Could you check a few things on this model? Use its own coordinates, in mm. Face numbers are marked on the shaded views. A direction names the side the tool comes from. Round coordinates to 2 decimals unless told otherwise and drop trailing zeros. Write each loop counter-clockwise with the first axis right and the second up, starting at its lowest first coordinate (ties: lowest second). Pieces come first, ordered by that corner, then holes. Notation, with made-up numbers: M 35.5,-24.75 L 44.5,-24.75 A22 ccw 44.5,5.25 Z; hole C 10,28 d1. An arc over 180 degrees is marked long. One line per item, written item: value. Start each with the question number.
(1) I'm going to push flat-ended pins straight in: pin 1 Ø10 at (x, z) = (-22.5, -3) entering from -Y; pin 2 Ø10 at (x, y) = (43, -3) entering from -Z; pin 3 Ø5 at (x, z) = (45.5, -7) entering from -Y. Where does each tip first touch, or does it pass through?
(2) Which directions (+Z, -Z, +X, -X, +Y, -Y) give clear straight access to the entire face, cutting with the end or side of a thin tool? Please do the marked faces 1 and 2.
(3) If I drill on L1, parallel to X at y = -8.5, z = -1.5; L2, parallel to Y at x = 54.5, z = 0; L3, parallel to X at y = -6.5, z = 0, over which ranges is the centre line in solid material (lowest first)?
(4) I want a section at A-A on x = 51.5. Please give me the cut outline in (y, z).
(5) I want a section at B-B on x = 32. Please give me the cut outline in (y, z).
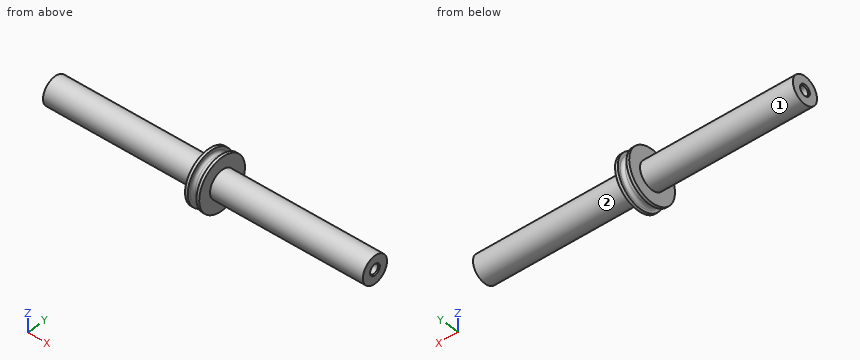
```python
from build123d import *

# Parameters (mm, degrees)
SKETCH1_W   = 1.5875
SKETCH1_H   = 7.5
SKETCH1_W_2 = 1
SKETCH1_H_2 = 9.5
SKETCH1_W_3 = 55.9125
SKETCH1_H_3 = 5
FILLET1_R   = 1


with BuildPart() as part:
    # Sketch1 → Revolve1 (revolve)
    with BuildSketch(Plane(origin=(0, 0, 0), x_dir=(1, 0, 0), z_dir=(0, 1, 0))):
        Polygon((-2.5875, 0), (-1.5875, 0), (-1.5875, 7.5), (-1.5875, 9.5), (-2.5875, 9.5), (-2.5875, 5), align=None)
        with Locations((-0.79375, 3.75)):
            Rectangle(SKETCH1_W, SKETCH1_H)
        with Locations((0.79375, 3.75)):
            Rectangle(SKETCH1_W, SKETCH1_H)
        with Locations((2.0875, 4.75)):
            Rectangle(SKETCH1_W_2, SKETCH1_H_2)
        with Locations((-30.54375, 2.5)):
            Rectangle(SKETCH1_W_3, SKETCH1_H_3)
        with Locations((30.54375, 2.5)):
            Rectangle(SKETCH1_W_3, SKETCH1_H_3)
    revolve(axis=Axis((-2.646790194, 0, 0), (1, 0, 0)))

    # Fillet1
    fillet1_edges = [part.edges().sort_by_distance(p)[0] for p in [
        (-1.5875, 0, 7.5),
        (1.5875, 0, 7.5),
    ]]
    fillet(fillet1_edges, radius=FILLET1_R)

    # Sketch3 → M4x0.7 Tapped Hole1 (revolve, cut)
    with BuildSketch(Plane(origin=(-58.5, 0, 0), x_dir=(0, 0, 1), z_dir=(0, 1, 0))):
        Polygon((0, 0), (0, 15.991420021), (1.65, 15), (1.65, 0.375), (2.025, 0), align=None)
    m4x0_7_tapped_hole1 = revolve(axis=Axis((-64.85, 0, 0), (1, 0, 0)), mode=Mode.SUBTRACT)

    # Mirror1: M4x0.7 Tapped Hole1 across plane
    add(m4x0_7_tapped_hole1.mirror(Plane(origin=(0, 0, 0), x_dir=(0, 0, 1), z_dir=(1, 0, 0))), mode=Mode.SUBTRACT)


solid = part.part
```
Found:
1. pin 1: stops at y = -5
1. pin 2: stops at z = -5
1. pin 3: stops at y = -2.18
2. face 1: -X
2. face 2: +X
3. L1: x = -2.59 to -1.59, 1.59 to 2.59
3. L2: y = -5 to -1.65, 1.65 to 5
3. L3: x = -2.59 to 2.59
4. outline: C 0,0 d10; hole C 0,0 d3.3
5. outline: C 0,0 d10
